```python
from build123d import *

# Parameters (mm, degrees)
CUT_EXTRUDE1_DEPTH = 0.875
FILLET1_R          = 0.4
FILLET2_R          = 1


with BuildPart() as part:
    # Sketch1 → Revolve1 (revolve)
    with BuildSketch(Plane(origin=(0, 0, 0), x_dir=(0, 0, -1), z_dir=(1, 0, 0)), mode=Mode.PRIVATE) as revolve1_sk:
        Polygon((-1.3125, 3), (0, 1.5), (10.628679656, 1.5), (14.25, 0), (-1.75, 0), (-1.75, 3), align=None)
    revolve(revolve1_sk.sketch.rotate(Axis((0, 0, 94.243212435), (0, 0, -1)), 90), axis=Axis((0, 0, 94.243212435), (0, 0, -1)))

    # Sketch5 → Cut-Extrude1 (cut)
    with BuildSketch(Plane.XY.offset(1.75)):
        Polygon((0, 1.8), (-0.36, 1.8), (-0.36, 0.36), (-1.8, 0.36), (-1.8, 0), (-1.8, -0.36), (-0.36, -0.36), (-0.36, -1.8), (0, -1.8), (0.36, -1.8), (0.36, -0.36), (1.8, -0.36), (1.8, 0), (1.8, 0.36), (0.36, 0.36), (0.36, 1.8), align=None)
    extrude(amount=-CUT_EXTRUDE1_DEPTH, mode=Mode.SUBTRACT)

    # Fillet1
    fillet1_edges = [part.edges().sort_by_distance(p)[0] for p in [
        (-1.5, 0, 0),
    ]]
    fillet(fillet1_edges, radius=FILLET1_R)

    # Fillet2
    fillet2_edges = [part.edges().sort_by_distance(p)[0] for p in [
        (-1.5, 0, -10.628679656),
    ]]
    fillet(fillet2_edges, radius=FILLET2_R)


solid = part.part
```
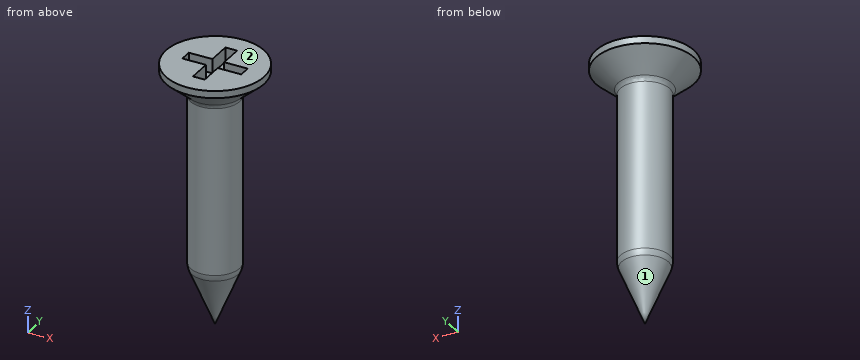
The model under review builds one solid part; all positions refer to its coordinate system, in mm. Face numbers are marked on the shaded views. Round coordinates to 2 decimals unless told otherwise and drop trailing zeros. Order: outer loops, then holes, each group sorted by start corner. A loop starts at its lowest first (then second) coordinate and runs counter-clockwise, first axis right, second up. Notation, with made-up numbers: (62.5, 86) -> (105.5, 86) arc R19 cw to (105.5, 107) -> close; hole circle Ø8 at (51.5, 71.25). An arc over 180 degrees is marked (long way). One line per item, written item: value. Start each with the question number.
Q1. Clearance check with flat-ended pins moving along their axes: pin 1 Ø0.7 at (y, z) = (-1, 1.5) entering from +X; pin 2 Ø3 at (x, y) = (-1, -2) entering from -Z; pin 3 Ø3 at (y, z) = (-0.5, -4.5) entering from +X. State where each tip first meets the part, or that it passes through.
Q2. Mouldability with a two-part tool opening along Y and no side actions: class the marked faces 1 and 2 as released by +Y, released by -Y, zero draft, split by the parting line, or undercut.
Q3. Take a section at A-A (z = -4). Write out the cut boundary in (x, y).
Q4. Wall thickness on line 1 (Z direction, x = -1.5, y = -2) (3 decimals); line 2 (X direction, y = 1.5, z = 0.5); line 3 (X direction, y = 1, z = -2.5): over which ranges is each line inside the solid? List them lowest first.
Reported:
1. pin 1: stops at x = 2.93
1. pin 2: stops at z = -12.47
1. pin 3: stops at x = 1.5
2. face 1: split by the parting line
2. face 2: zero draft
3. outline: circle Ø3 at (0, 0)
4. line 1: z = 0.875 to 1.75
4. line 2: x = -1.43 to 1.43
4. line 3: x = -1.12 to 1.12
